Here's how the part is built. I have some questions about the finished solid (model axes, mm). Coordinates: 2 decimals unless noted, no trailing zeros. Answer in a Markdown table with one row per item. Add a question column.
Item 1: If I drill on line 1 along X through (y, z) = (9, 3); line 2 along Y through (x, z) = (12, 9.75), over which ranges is the centre line in solid material (lowest first)? Write a range as from..to.
Item 2: Thinking about a two-plate mould opening in X: for faces 1 (the flat face through (-1, 1, 0)), 2 (the cylindrical face through (-9.675, -12.398, 6.439)), 3 (the flat face through (-38.1, 1, 6)), which applies, +X half, -X half, draft (parallel to the pull), parting line (faces both ways), or undercut?
Item 3: Will these pins go through, and if not, where does the flat tip stop? pin 1 Ø5 at (x, y) = (-10, 12.5) entering from -Z; pin 2 Ø2.5 at (x, y) = (10.61, -10.61) entering from +Z.
```python
from build123d import *

# Parameters (mm, degrees)
BOSS_EXTRUDE1_DEPTH = 12.7
SKETCH2_R           = 2.0193
CUT_EXTRUDE1_DEPTH  = 56.358016583


with BuildPart() as part:
    # Sketch1 → Boss-Extrude1 (new body)
    with BuildSketch(Plane.XY):
        Polygon((-38.1, 38.1), (-38.1, -38.1), (-12.7, -38.1), (12.7, -38.1), (38.1, -38.1), (38.1, 38.1), (12.7, 38.1), (-12.7, 38.1), align=None)
    extrude(amount=BOSS_EXTRUDE1_DEPTH)

    # Sketch2 → Cut-Extrude1 (cut, through all)
    with BuildSketch(Plane.XY.offset(12.7)):
        with Locations((10.606601718, 10.606601718)):
            Circle(SKETCH2_R)
        with Locations(Location((10.606601718, -10.606601718, 0), (0, 0, 180))):
            Circle(SKETCH2_R)
        with Locations((-10.606601718, -10.606601718)):
            Circle(SKETCH2_R)
        with Locations(Location((-10.606601718, 10.606601718, 0), (0, 0, 180))):
            Circle(SKETCH2_R)
    extrude(amount=-CUT_EXTRUDE1_DEPTH, mode=Mode.SUBTRACT)


solid = part.part
```
Values follow:
| question | item | result |
|---|---|---|
| 1 | line 1 | x = -38.1..-11.83, -9.38..9.38, 11.83..38.1 |
| 1 | line 2 | y = -38.1..-12.07, -9.15..9.15, 12.07..38.1 |
| 2 | face 1 | draft |
| 2 | face 2 | undercut |
| 2 | face 3 | -X half |
| 3 | pin 1 | stops at z = 0 |
| 3 | pin 2 | passes through |
